```python
from build123d import *

# Parameters (mm, degrees)
F0_R     = 25.4
F1_DEPTH = 3.429


with BuildPart() as f1:
    # F0 (on Front) → F1 (new body)
    with BuildSketch(Plane.XZ):
        Polygon((644.354287, -53.912491), (644.354287, -71.692491), (647.529287, -71.692491), (647.529287, -112.014991), (887.051287, -115.189991), (887.051287, -73.914991), (883.876287, -73.914991), (883.876287, -54.864991), (887.051287, -54.864991), (887.051287, -13.589991), (817.836287, -13.589991), (817.836287, -16.764991), (798.786287, -16.764991), (798.786287, -13.589991), (735.794287, -13.589991), (735.794287, -16.764991), (716.744287, -16.764991), (716.744287, -13.589991), (647.529287, -13.589991), (647.529287, -53.912491), align=None)
        with Locations((697.595912, -62.823446)):
            Circle(F0_R, mode=Mode.SUBTRACT)
        with Locations((767.482107, -62.823446)):
            Circle(F0_R, mode=Mode.SUBTRACT)
        with Locations((837.082629, -62.823446)):
            Circle(F0_R, mode=Mode.SUBTRACT)
    extrude(amount=F1_DEPTH)


solid = f1.part
```
CAD build for the part. Positions are in the model's coordinates, mm. Coordinates: 2 decimals unless noted, no trailing zeros. Order: outer loops, then holes, each group sorted by start corner. A loop starts at its lowest first (then second) coordinate and runs counter-clockwise, first axis right, second up. Notation, with made-up numbers: M 13,76.5 L 65,76.5 A16 cw 65,97.5 Z; hole C 32.25,32 d9. An arc over 180 degrees is marked long. Answer as CSV lines item,"result".
1) Drill centre lines: L1, parallel to X at y = -2.75, z = -42; L2, parallel to X at y = -1.6, z = -74.5; L3, parallel to X at y = -2.9, z = -95. Where is each one in solid material? Low to high. Write a range as from..to.
Verdict:
L1,"647.53..683.05, 712.14..752.94, 782.03..822.54, 851.63..887.05"
L2,"647.53..675.04, 720.15..744.93, 790.04..814.53, 859.64..887.05"
L3,"647.53..887.05"
2) Cut at A-A (x = 776). List the corners of the cut face in (y, z).
Verdict:
outline,"M -3.43,-113.72 L 0,-113.72 L 0,-86.75 L -3.43,-86.75 Z; M -3.43,-38.89 L 0,-38.89 L 0,-13.59 L -3.43,-13.59 Z"
3) Mould opens along Z. For faces 1 (the cylindrical face through (742.107, -1.69, -61.707)), 2 (the flat face through (737, 0, -64)) say: released by +Z, released by -Z, zero draft, split by the parting line, or undercut.
Verdict:
face 1,"undercut"
face 2,"zero draft"
4) Cut at D-D (x = 700.5). List the corners of the cut face in (y, z).
Verdict:
outline,"M -3.43,-112.72 L 0,-112.72 L 0,-88.06 L -3.43,-88.06 Z; M -3.43,-37.59 L 0,-37.59 L 0,-13.59 L -3.43,-13.59 Z"
5) Cut at C-C (y = -2.1). List the corners of the cut face in (x, z) (1 decimal).
Verdict:
outline,"M 644.4,-71.7 L 647.5,-71.7 L 647.5,-112 L 887.1,-115.2 L 887.1,-73.9 L 883.9,-73.9 L 883.9,-54.9 L 887.1,-54.9 L 887.1,-13.6 L 817.8,-13.6 L 817.8,-16.8 L 798.8,-16.8 L 798.8,-13.6 L 735.8,-13.6 L 735.8,-16.8 L 716.7,-16.8 L 716.7,-13.6 L 647.5,-13.6 L 647.5,-53.9 L 644.4,-53.9 Z; hole C 697.6,-62.8 d50.8; hole C 767.5,-62.8 d50.8; hole C 837.1,-62.8 d50.8"
6) Cut at B-B (z = -82). List the corners of the cut face in (x, y), then the cut area to 3 significant figures.
Verdict:
outline,"M 647.53,-3.43 L 680.94,-3.43 L 680.94,0 L 647.53,0 Z; M 714.25,-3.43 L 750.83,-3.43 L 750.83,0 L 714.25,0 Z; M 784.14,-3.43 L 820.43,-3.43 L 820.43,0 L 784.14,0 Z; M 853.74,-3.43 L 887.05,-3.43 L 887.05,0 L 853.74,0 Z"
area,"479 mm2"
7) Flat gauge pins, fed straight in: P1, Ø1.6, axis at x = 646.5, y = -2, coming from the +Z side; P2, Ø1, axis at x = 646, y = -1, coming from the -Z side; P3, Ø1.6, axis at x = 885, y = -1.5, coming from the -Z side. Where does each tip first touch, or does it go through?
Verdict:
P1,"z = -53.91"
P2,"z = -71.69"
P3,"z = -115.17"
